Build history of the part. All positions in model axes, mm. A direction names the side the tool comes from. Give positions to 0.01 mm unless a question says otherwise; leave off trailing zeros. Write each loop counter-clockwise with the first axis right and the second up, starting at its lowest first coordinate (ties: lowest second). Pieces come first, ordered by that corner, then holes. Notation, with made-up numbers: M 1.5,72 L 23.5,72 A15 ccw 23.5,99 Z; hole C 89,12 d1. An arc over 180 degrees is marked long. Return JSON: item names as keys, results as strings. Group by question number.
Q1. Pull direction Y, two halves, no side cores. Call faces 3 (the flat face through (3, -42, -15.875)), 4 (the flat face through (3, -1, 38.1)), 5 (the flat face through (3, -57.15, 0)), 6 (the cylindrical face through (3.22, 55.34, -36.19)): +Y half, -Y half, draft (parallel to the pull), parting line (faces both ways), or undercut.
Q2. Band-saw the part on B-B, the plane x = 2. Count the separate pieces of the cut face and the enclosed holes in it, then the cut area to 3 significant figures.
Q3. Band-saw the part on A-A, the plane y = 42. Give the cut face in (x, z) (3 decimals).
Q4. Tool access for faces 1 (the flat face through (0, 1, 1)), 2 (the flat face through (3, 42, 15.875)): list every direction of +Z, -Z, +X, -X, +Y, -Y with a clear straight run to the whole face (end or side of a thin tool).
Q5. Wall check: probe 1 along Z at (x, y) = (0.5, 36) (3 decimals); probe 2 along Z at (x, y) = (0.5, 24); probe 3 along Y at (x, z) = (4, 18). Give the ranges that are in metal, low to high.
from build123d import *

# Parameters (mm, degrees)
SKETCH1_W               = 76.2
SKETCH1_H               = 114.3
BOSS_EXTRUDE1_DEPTH     = 6.35
F_1_4_20_TAPPED_HOLE1_D = 5.1054
CUT_EXTRUDE1_DEPTH      = 69.978656119
FILLET1_R               = 6.35


with BuildPart() as part:
    # Sketch1 → Boss-Extrude1 (new body)
    with BuildSketch(Plane(origin=(0, 0, 0), x_dir=(0, 0, -1), z_dir=(1, 0, 0))):
        Rectangle(SKETCH1_W, SKETCH1_H)
    extrude(amount=BOSS_EXTRUDE1_DEPTH)

    # 1/4-20 Tapped Hole1 (through all)
    with Locations(Plane(origin=(6.35, 0, 0), x_dir=(0, 0, -1), z_dir=(1, 0, 0))):
        with Locations((-20.6375, 21.9075), (20.6375, 21.9075), (20.6375, -21.9075), (-20.6375, -21.9075)):
            Hole(F_1_4_20_TAPPED_HOLE1_D / 2)

    # Sketch4 → Cut-Extrude1 (cut, through all)
    with BuildSketch(Plane(origin=(6.35, 0, 0), x_dir=(0, 0, -1), z_dir=(1, 0, 0))):
        with BuildLine():
            Line((15.875, 49.022), (15.875, 35.052))
            ThreePointArc((15.875, 35.052), (19.05, 31.877), (22.225, 35.052))
            Line((22.225, 35.052), (22.225, 49.022))
            ThreePointArc((22.225, 49.022), (19.05, 52.197), (15.875, 49.022))
        make_face()
        with BuildLine():
            Line((-22.225, 49.022), (-22.225, 35.052))
            ThreePointArc((-22.225, 35.052), (-19.05, 31.877), (-15.875, 35.052))
            Line((-15.875, 35.052), (-15.875, 49.022))
            ThreePointArc((-15.875, 49.022), (-19.05, 52.197), (-22.225, 49.022))
        make_face()
        with BuildLine():
            Line((-15.875, -49.022), (-15.875, -35.052))
            ThreePointArc((-15.875, -35.052), (-19.05, -31.877), (-22.225, -35.052))
            Line((-22.225, -35.052), (-22.225, -49.022))
            ThreePointArc((-22.225, -49.022), (-19.05, -52.197), (-15.875, -49.022))
        make_face()
        with BuildLine():
            Line((22.225, -49.022), (22.225, -35.052))
            ThreePointArc((22.225, -35.052), (19.05, -31.877), (15.875, -35.052))
            Line((15.875, -35.052), (15.875, -49.022))
            ThreePointArc((15.875, -49.022), (19.05, -52.197), (22.225, -49.022))
        make_face()
    extrude(amount=-CUT_EXTRUDE1_DEPTH, mode=Mode.SUBTRACT)

    # Fillet1
    fillet1_edges = [part.edges().sort_by_distance(p)[0] for p in [
        (3.175, -57.15, -38.1),
        (3.175, -57.15, 38.1),
        (3.175, 57.15, 38.1),
        (3.175, 57.15, -38.1),
    ]]
    fillet(fillet1_edges, radius=FILLET1_R)


solid = part.part
From the geometry:
{
 "1": {"face 3": "undercut", "face 4": "draft", "face 5": "-Y half", "face 6": "+Y half"},
 "2": {"separate pieces": "1", "enclosed holes": "8", "area": "8,110 mm^2"},
 "3": {"outline": "M 0,-38.1 L 6.35,-38.1 L 6.35,-22.225 L 0,-22.225 Z; M 0,-15.875 L 6.35,-15.875 L 6.35,15.875 L 0,15.875 Z; M 0,22.225 L 6.35,22.225 L 6.35,38.1 L 0,38.1 Z"},
 "4": {"face 1": "+Z, -Z, -X, +Y, -Y", "face 2": "+X, -X"},
 "5": {"probe 1": "z = -38.1 to -22.225, -15.875 to 15.875, 22.225 to 38.1", "probe 2": "z = -38.1 to -22.1, -19.18 to 19.18, 22.1 to 38.1", "probe 3": "y = -57.15 to -52.02, -32.06 to 32.06, 52.02 to 57.15"}
}
